```python
from build123d import *

# Parameters (mm, degrees)
SKETCH1_W               = 30
SKETCH1_H               = 15
BOSS_EXTRUDE1_DEPTH     = 5.5
CUT_EXTRUDE2_DEPTH      = 18.649362595
CUT_EXTRUDE2_DEPTH_BACK = 18.649362595
SKETCH2_W               = 0.5
SKETCH2_H               = 0.2
FILLET1_R               = 1


with BuildPart() as part:
    # Sketch1 → Boss-Extrude1 (new body)
    with BuildSketch(Plane(origin=(0, 0, 0), x_dir=(1, 0, 0), z_dir=(0, 1, 0))):
        Rectangle(SKETCH1_W, SKETCH1_H)
    extrude(amount=BOSS_EXTRUDE1_DEPTH)

    # Sketch2 → Cut-Extrude2 (cut, two sides: drawn at the far end of the back side and taken through both)
    with BuildSketch(Plane(origin=(0, 0, 0), x_dir=(0, 0, -1), z_dir=(1, 0, 0)).offset(-CUT_EXTRUDE2_DEPTH_BACK)):
        with Locations((-5.75, 5.4)):
            Rectangle(SKETCH2_W, SKETCH2_H)
        with Locations((-3.75, 5.4)):
            Rectangle(SKETCH2_W, SKETCH2_H)
        with Locations((-1.75, 5.4)):
            Rectangle(SKETCH2_W, SKETCH2_H)
        with Locations((0.25, 5.4)):
            Rectangle(SKETCH2_W, SKETCH2_H)
        with Locations((2.25, 5.4)):
            Rectangle(SKETCH2_W, SKETCH2_H)
        with Locations((4.25, 5.4)):
            Rectangle(SKETCH2_W, SKETCH2_H)
        with Locations((6.25, 5.4)):
            Rectangle(SKETCH2_W, SKETCH2_H)
    extrude(amount=CUT_EXTRUDE2_DEPTH + CUT_EXTRUDE2_DEPTH_BACK, mode=Mode.SUBTRACT)

    # Sketch8 → Cut-Revolve1 (revolve, cut)
    with BuildSketch(Plane.XY.offset(4), mode=Mode.PRIVATE) as cut_revolve1_sk:
        Polygon((10.25, 0), (10.25, 3), (9, 3.721687836), (9, 0), align=None)
    cut_revolve1 = revolve(cut_revolve1_sk.sketch.rotate(Axis((9, 0, 4), (0, 1, 0)), 90), axis=Axis((9, 0, 4), (0, 1, 0)), mode=Mode.SUBTRACT)

    # Mirror1: Cut-Revolve1 across plane
    add(cut_revolve1.mirror(Plane.XY), mode=Mode.SUBTRACT)

    # Mirror2: Cut-Revolve1 across plane
    add(cut_revolve1.mirror(Plane(origin=(0, 0, 0), x_dir=(0, 0, 1), z_dir=(1, 0, 0))), mode=Mode.SUBTRACT)

    # Mirror2 copy 1 sketch → Mirror2 copy 1 (revolve, cut)
    with BuildSketch(Plane(origin=(0, 0, -4), x_dir=(-1, 0, 0), z_dir=(0, 0, -1))):
        Polygon((10.25, 0), (10.25, 3), (9, 3.721687836), (9, 0), align=None)
    revolve(axis=Axis((-9, 0, -4), (0, 1, 0)), mode=Mode.SUBTRACT)

    # Sketch9 → Cut-Revolve2 (revolve, cut)
    with BuildSketch(Plane.XY, mode=Mode.PRIVATE) as cut_revolve2_sk:
        Polygon((-15, 2.5), (-7.678312164, 2.5), (-8.4, 3.75), (-15, 3.75), align=None)
    revolve(cut_revolve2_sk.sketch.rotate(Axis((-15, 2.5, 0), (-1, 0, 0)), 180), axis=Axis((-15, 2.5, 0), (-1, 0, 0)), mode=Mode.SUBTRACT)

    # Fillet1
    fillet1_edges = [part.edges().sort_by_distance(p)[0] for p in [
        (-15, 2.75, -7.5),
        (15, 2.75, -7.5),
        (15, 2.75, 7.5),
        (-15, 2.75, 7.5),
    ]]
    fillet(fillet1_edges, radius=FILLET1_R - 0.0001)  # a hair under: the kernel refuses the full size


solid = part.part
```
Design review of the part built by this model. Coordinates are the model's own, in mm. A direction names the side the tool comes from. Coordinates: 2 decimals unless noted, no trailing zeros. Write each loop counter-clockwise with the first axis right and the second up, starting at its lowest first coordinate (ties: lowest second). Pieces come first, ordered by that corner, then holes.
1) Add section A-A (y = 0.5). Write out the cut boundary in (x, z), plus the area to 3 significant figures.
2) Add section B-B (y = 2.2). State how many separate pieces and enclosed holes the cut face has, plus the area to 3 significant figures.
3) Mouldability with a two-part tool opening along X and no side actions: class faces 1 (the cylindrical face through (-14.715, 2.788, -7.199)), 2 (the cylindrical face through (8.95, 1.52, 5.25)), 3 (the flat face through (0, 0, 0)), 4 (the cylindrical face through (-8.95, 1.52, 5.25)) as +X half, -X half, draft (parallel to the pull), parting line (faces both ways), or undercut.
4) Machinability: for faces 5 (the cylindrical face through (-8.01, 1.52, -4.76)), 6 (the cylindrical face through (-11.75, 1.31, 0.38)), 7 (the cylindrical face through (-14.715, 2.788, 7.199)), which of the approach directions +Z, -Z, +X, -X, +Y, -Y give a long, thin tool a straight path to every point of the face, cutting with its end or side? Answer none if there is none.
5) To check wall thickness, follow L1, parallel to X at y = 0.8, z = 4; L2, parallel to X at y = 2.25, z = 3.5; L3, parallel to Z at x = 9.5, y = 2.25. State the ranges of each line that lie inside material, in increasing order.
6) Insertion check: pin 1 (1.5 mm diameter, centred on y = 2.5, z = 0, fed in from -X); pin 2 (1.5 mm diameter, centred on x = 0.5, z = -0.5, fed in from -Y). Each pin has a flat end and moves straight along its axis. Give the tip position at first contact, or say it passes through.
Check result:
1. outline: (-15, -6.5) arc R1 ccw to (-14, -7.5) - (14, -7.5) arc R1 ccw to (15, -6.5) - (15, 6.5) arc R1 ccw to (14, 7.5) - (-14, 7.5) arc R1 ccw to (-15, 6.5) - close; hole circle Ø2.5 at (-9, -4); hole circle Ø2.5 at (-9, 4); hole circle Ø2.5 at (9, -4); hole circle Ø2.5 at (9, 4)
1. area: 430 mm2
2. separate pieces: 1
2. enclosed holes: 4
2. area: 413 mm2
3. face 1: -X half
3. face 2: undercut
3. face 3: draft
3. face 4: undercut
4. face 5: -Y
4. face 6: -X
4. face 7: +Z, -X, +Y, -Y
5. L1: x = -15 to -10.25, -7.75 to 7.75, 10.25 to 15
5. L2: x = -15 to -10.15, -7.85 to 7.85, 10.15 to 15
5. L3: z = -7.5 to -5.15, -2.85 to 2.85, 5.15 to 7.5
6. pin 1: stops at x = -8.11
6. pin 2: stops at y = 0
